Here's how the part is built. I have some questions about the finished solid (model axes, mm). Face numbers are marked on the shaded views. A direction names the side the tool comes from. Round coordinates to 2 decimals unless told otherwise and drop trailing zeros. Write each loop counter-clockwise with the first axis right and the second up, starting at its lowest first coordinate (ties: lowest second). Pieces come first, ordered by that corner, then holes. Notation, with made-up numbers: (-32, -12) -> (13, -12) arc R4 ccw to (13, -8) -> close; hole circle Ø3 at (83.25, -5). An arc over 180 degrees is marked (long way). Answer as CSV lines item,"result".
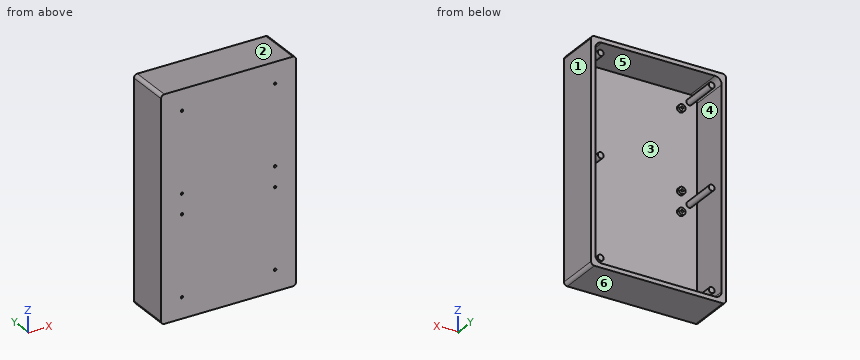
Autodesk Inventor part; units mm, degrees
ref_plane "YZ Plane" through (0, 0, 0) normal (1, 0, 0) x (0, 1, 0)
ref_plane "XZ Plane" through (0, 0, 0) normal (0, 1, 0) x (-1, 0, 0)
ref_plane "XY Plane" through (0, 0, 0) normal (0, 0, 1) x (1, 0, 0)
sketch "Sketch1" plane through (0, 0, 0) normal (0, 1, 0) x (-1, 0, 0)
  line L0 (3.175, 0) -> (125.603, 0)
  line L1 (128.778, -3.175) -> (128.778, -208.153)
  line L2 (125.603, -211.328) -> (3.175, -211.328)
  line L3 (0, -208.153) -> (0, -3.175)
  line L4 (10.414, -4.064) -> (118.364, -4.064)
  line L5 (124.714, -10.414) -> (124.714, -200.914)
  line L6 (118.364, -207.264) -> (10.414, -207.264)
  line L7 (4.064, -200.914) -> (4.064, -10.414)
  circle A0 centre (117.348, -11.43) radius 2.794
  circle A1 centre (11.43, -11.43) radius 2.794
  circle A2 centre (117.348, -105.664) radius 2.794
  circle A3 centre (11.43, -105.664) radius 2.794
  circle A4 centre (117.348, -199.898) radius 2.794
  circle A5 centre (11.43, -199.898) radius 2.794
  line L8 (124.714, -105.664) -> (4.064, -105.664)
  line L9 (64.389, -4.064) -> (64.389, -207.264)
  circle A6 centre (108.839, -19.939) radius 1.143
  circle A7 centre (108.839, -19.939) radius 3.302
  circle A8 centre (108.839, -96.139) radius 3.302
  circle A9 centre (108.839, -96.139) radius 1.143
  circle A10 centre (19.939, -19.939) radius 3.302
  circle A11 centre (19.939, -19.939) radius 1.143
  circle A12 centre (19.939, -96.139) radius 3.302
  circle A13 centre (19.939, -96.139) radius 1.143
  circle A14 centre (108.839, -191.389) radius 1.143
  circle A15 centre (108.839, -191.389) radius 3.302
  circle A16 centre (108.839, -115.189) radius 3.302
  circle A17 centre (108.839, -115.189) radius 1.143
  circle A18 centre (19.939, -191.389) radius 3.302
  circle A19 centre (19.939, -191.389) radius 1.143
  circle A20 centre (19.939, -115.189) radius 3.302
  circle A21 centre (19.939, -115.189) radius 1.143
  arc A22 (128.778, -3.175) -> (125.603, 0) centre (125.603, -3.175) ccw
  arc A23 (125.603, -211.328) -> (128.778, -208.153) centre (125.603, -208.153) ccw
  arc A24 (0, -208.153) -> (3.175, -211.328) centre (3.175, -208.153) ccw
  arc A25 (3.175, 0) -> (0, -3.175) centre (3.175, -3.175) ccw
  arc A26 (10.414, -4.064) -> (4.064, -10.414) centre (10.414, -10.414) ccw
  arc A27 (124.714, -10.414) -> (118.364, -4.064) centre (118.364, -10.414) ccw
  arc A28 (118.364, -207.264) -> (124.714, -200.914) centre (118.364, -200.914) ccw
  arc A29 (4.064, -200.914) -> (10.414, -207.264) centre (10.414, -200.914) ccw
  point P0 (0, 0)
  point P1 (128.778, -211.328)
  point P2 (128.778, 0)
  point P3 (0, -211.328)
  dimension "d0" = 128.778
  dimension "d1" = 211.328
  dimension "d2" = 203.2
  dimension "d3" = 120.65
  dimension "d4" = 4.064
  dimension "d5" = 4.064
  dimension "d6" = 5.588
  dimension "d9" = 105.918
  dimension "d12" = 94.234
  dimension "d15" = 0
  dimension "d16" = 52.959
  dimension "d17" = 2.286
  dimension "d18" = 6.604
  dimension "d21" = 76.2
  dimension "d24" = 88.9
  dimension "d27" = 44.45
  dimension "d28" = 9.525
  dimension "d29" = 3.175
  dimension "d30" = 6.35
  dimension "d31" = 6.35
extrude "Extrusion1" add sketch "Sketch1" along normal blind 3.556 contours L4 L9 L8 A3 L7 A26 | L4 A27 L5 L8 A2 L9 | L9 L6 A29 L7 L8 A3 | L8 A2 L5 A28 L6 L9
extrude "Extrusion2" add sketch "Sketch1" along normal blind 6.35 contours A7 | A8 | A10 | A12 | A15 | A16 | A18 | A20
extrude "Extrusion3" add sketch "Sketch1" along normal blind 38.1 contours L8 A2 | A2 L8 | L8 A3 | A3 L8 | A0 | A1 | A4 | A5
extrude "Extrusion4" add sketch "Sketch1" along normal blind 41.656 contours L0 A22 L1 A23 L2 A24 L3 A25
properties part number "Box"
1. Suppose I cut it at A-A on y = 31. Please give me the cut outline in (x, z) (3 decimals).
Numbers:
outline,"(-128.778, -208.153) arc R3.175 ccw to (-125.603, -211.328) -> (-3.175, -211.328) arc R3.175 ccw to (0, -208.153) -> (0, -3.175) arc R3.175 ccw to (-3.175, 0) -> (-125.603, 0) arc R3.175 ccw to (-128.778, -3.175) -> close; circle Ø5.588 at (-117.348, -199.898); circle Ø5.588 at (-117.348, -105.664); circle Ø5.588 at (-117.348, -11.43); circle Ø5.588 at (-11.43, -199.898); circle Ø5.588 at (-11.43, -105.664); circle Ø5.588 at (-11.43, -11.43); hole (-124.714, -200.914) arc R6.35 ccw to (-118.364, -207.264) -> (-10.414, -207.264) arc R6.35 ccw to (-4.064, -200.914) -> (-4.064, -10.414) arc R6.35 ccw to (-10.414, -4.064) -> (-118.364, -4.064) arc R6.35 ccw to (-124.714, -10.414) -> close"
2. Suppose I cut it at C-C on z = -77. Please give me the cut outline in (x, y), and give its area (3 significant figures).
Numbers:
outline,"(-128.78, 0) -> (0, 0) -> (0, 41.66) -> (-4.06, 41.66) -> (-4.06, 3.56) -> (-124.71, 3.56) -> (-124.71, 41.66) -> (-128.78, 41.66) -> close"
area,"768 mm^2"
3. On a 3-axis mill with a long thin cutter (end or side, diameter ignored), from which of +Z, -Z, +X, -X, +Y, -Y can I reach the whole of each face in a straight line? I mean the marked faces 5 and 6. Say none if no direction works.
Numbers:
face 5,"+Y"
face 6,"-Z, +X, -X, +Y, -Y"
4. If I drill on line 1 (X direction, y = 34.5, z = -21); line 2 (Z direction, x = -102, y = 7); line 3 (X direction, y = 5.5, z = -118), over which ranges is the centre line in solid material (lowest first)?
Numbers:
line 1,"x = -128.78 to -124.71, -4.06 to 0"
line 2,"z = -211.33 to -207.26, -4.06 to 0"
line 3,"x = -128.78 to -124.71, -110.57 to -107.11, -21.67 to -18.21, -4.06 to 0"
5. Suppose I cut it at B-B on x = -46. Please give me the cut outline in (y, z).
Numbers:
outline,"(0, -211.33) -> (41.66, -211.33) -> (41.66, -207.26) -> (3.56, -207.26) -> (3.56, -4.06) -> (41.66, -4.06) -> (41.66, 0) -> (0, 0) -> close"
6. If we mould it in two halves opening along Z, with no side actions, what happens to the marked faces 1, 2, 3 and 4? For each: released by +Z, released by -Z, zero draft, split by the parting line, or undercut.
Numbers:
face 1,"zero draft"
face 2,"released by +Z"
face 3,"undercut"
face 4,"undercut"
7. For pin 1 Ø5.5 at (x, z) = (-108.5, -95.5) entering from +Y; pin 2 Ø5 at (x, z) = (-16, -71) entering from +Y; pin 3 Ø6 at (x, z) = (-118.5, -199) entering from +Y; pin 4 Ø1.4 at (x, z) = (-19.939, -191.389) entering from +Y, each with a flat end and sliding along its axis, tell me the tip position at first contact or that it passes through.
Numbers:
pin 1,"stops at y = 6.35"
pin 2,"stops at y = 3.56"
pin 3,"stops at y = 38.1"
pin 4,"passes through"
